Could you check a few things on this drawing? It's one solid part, dimensions in mm from its lowest x, y, z. A direction names the side the tool comes from. Round coordinates to 2 decimals unless told otherwise and drop trailing zeros. Loops run counter-clockwise (first coordinate to the right, second up) from the corner with the lowest first, then second, coordinate; pieces in that order, holes last. Notation, with made-up numbers: (53, 32) -> (98, 32) arc R20 ccw to (98, 55) -> close; hole circle Ø10 at (-40, 1). An arc over 180 degrees is marked (long way). Use one line per item in the form item = value. Start each with the question number.
Item 1: If we section it at B-B (z = 78.5): Write out the boundary of the cut face in (x, y) (1 decimal).
Item 2: For the marked faces 1 and 2, which set-ups out of +Z, -Z, +X, -X, +Y, -Y let a thin tool reach every point of the face, with its end or its side?
Item 3: If I drill on L1, parallel to Z at x = 116, y = 100; L2, parallel to Y at x = 78, z = 73; L3, parallel to X at y = 12, z = 37.5 (1 decimal), over which ranges is the centre line in solid material (lowest first)? Write a range as [from, to].
Item 4: I'm going to push flat-ended pins straight in: pin 1 Ø1.5 at (x, z) = (107, 36.5) entering from -Y; pin 2 Ø3 at (y, z) = (131.5, 16.5) entering from +X; pin 3 Ø1 at (x, z) = (76, 41.5) entering from -Y; pin 4 Ø1 at (x, y) = (69.5, 45.5) entering from -Z. Where does each tip first touch, or does it pass through?
Item 5: If we section it at A-A (z = 21): Write out the boundary of the cut face in (x, y), then the cut area to 3 significant figures.
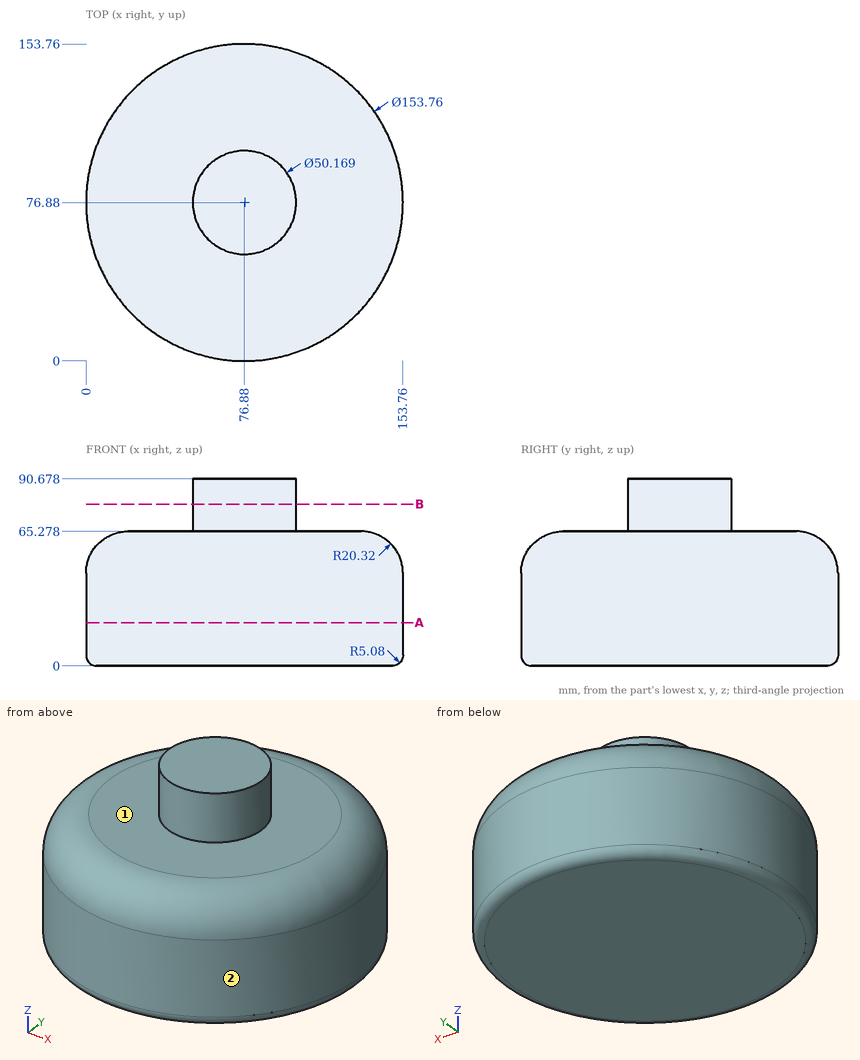
Values found:
q1.outline = circle Ø50.2 at (76.9, 76.9)
q2.face_1 = +Z
q2.face_2 = +Z, -Z
q3.L1 = [0, 65.28]
q3.L2 = [51.82, 101.94]
q3.L3 = [35.6, 118.1]
q4.pin_1 = 5.83
q4.pin_2 = 132.46
q4.pin_3 = 0
q4.pin_4 = 0
q5.outline = circle Ø153.76 at (76.88, 76.88)
q5.area = 18,600 mm2
